Source: CAD feature listing. Evaluate the final solid. Frame: model axes, mm. A direction names the side the tool comes from. Round coordinates to 2 decimals unless told otherwise and drop trailing zeros. Order: outer loops, then holes, each group sorted by start corner. A loop starts at its lowest first (then second) coordinate and runs counter-clockwise, first axis right, second up. Notation, with made-up numbers: (51.5, 78) -> (98.5, 78) arc R20 cw to (98.5, 91) -> close; hole circle Ø3 at (-7.75, -29). An arc over 180 degrees is marked (long way). Use a Markdown table: item, result. Add a question column.
Autodesk Inventor part; units mm, degrees
ref_plane "YZ Plane" through (0, 0, 0) normal (1, 0, 0) x (0, 1, 0)
ref_plane "XZ Plane" through (0, 0, 0) normal (0, 1, 0) x (-1, 0, 0)
ref_plane "XY Plane" through (0, 0, 0) normal (0, 0, 1) x (1, 0, 0)
sketch "草圖1" plane through (0, 0, 0) normal (0, 1, 0) x (-1, 0, 0)
  line L0 (0, 0) -> (-30, 0)
  line L1 (-30, 0) -> (-30, -50)
  line L2 (-30, -50) -> (0, -50)
  line L3 (0, -50) -> (0, 0)
  line L4 (-30, -50) -> (-60, -50)
  line L5 (-60, -50) -> (-60, -30)
  line L6 (-60, -30) -> (-30, -30)
  line L7 (-30, -30) -> (-30, -50)
  dimension "d0" = 30
  dimension "d1" = 20
  dimension "d2" = 30
  dimension "d6" = 30
extrude "擠出1" add sketch "草圖1" along normal blind 10
sketch "草圖2" plane through (60, 0, -50) normal (0, 0, -1) x (-1, 0, 0)
  line L0 (60, 0) -> (60, 10)
  line L1 (60, 10) -> (40, 10)
  line L2 (40, 10) -> (40, 30)
  line L3 (40, 30) -> (60, 30)
  line L4 (60, 30) -> (60, 10)
  line L5 (40, 10) -> (10, 10)
  line L6 (10, 10) -> (10, 20)
  line L7 (10, 20) -> (40, 20)
  line L8 (40, 20) -> (40, 10)
  line L9 (10, 10) -> (0, 10)
  line L10 (0, 10) -> (0, 50)
  line L11 (0, 50) -> (10, 50)
  line L12 (10, 50) -> (10, 10)
  dimension "d7" = 10
  dimension "d8" = 30
  dimension "d9" = 20
  dimension "d10" = 20
  dimension "d11" = 10
  dimension "d12" = 40
extrude "擠出2" add sketch "草圖2" against normal blind 10
sketch "草圖3" plane through (0, 0, -50) normal (-1, 0, 0) x (0, 0, 1)
  line L0 (0, 30) -> (10, 30)
  line L1 (50, 10) -> (20, 10)
  line L2 (10, 30) -> (50, 10)
  line L3 (50, 10) -> (10, 10)
  line L4 (10, 20) -> (10, 30)
  line L5 (10, 10) -> (10, 30)
  point P0 (50, 0)
extrude "擠出3" add sketch "草圖3" against normal blind 10
fillet "圓角1" radius 10 3 edges at (60, 50, -45) (60, 5, -30) (30, 5, 0)
properties part number "5"
1) Line query: probe 1 along Y at (x, z) = (24, -27); probe 2 along Y at (x, z) = (11.5, -43.5). Output: solid intervals per line, ascending. Write a range as from..to.
2) Section D-D on y = 17. Output: boundary loops of the cut face in (x, z), then the cut area to 3 significant figures.
3) Section C-C on x = 38.5. Output: boundary loops of the cut face in (y, z), then the cut area to 3 significant figures.
4) Draft query along X for faces 4 (the flat face through (10, 16, -29)), 5 (the flat face through (10, 5, 0)), 6 (the flat face through (50, 35, -45)). Return one class per face: pulls with the +X half, pulls with the -X half, needs draft (parallel to the pull), parting line crosses it, or undercut.
5) Section A-A on y = 25. Output: boundary loops of the cut face in (x, z).
6) First-contact query: pin 1 Ø8 at (y, z) = (34.5, -45.5) entering from -X; pin 2 Ø6 at (x, y) = (29, 17) entering from +Z; pin 3 Ø10 at (y, z) = (20.5, -25.5) entering from +X. Flat tips, straight axial feed; report the tip coordinate or a pass-through.
7) Reachability of faces 1 (the flat face through (35, 20, -45)), 2 (the flat face through (41, 17, -40)), 3 (the flat face through (30, 5, -20)) from +Z, -Z, +X, -X, +Y, -Y: full face, straight path, thin tool, end or side. Return the list, or none.
Conclusion:
| question | item | result |
|---|---|---|
| 1 | probe 1 | y = 0..10 |
| 1 | probe 2 | y = 0..30 |
| 2 | outline | (0, -50) -> (60, -50) -> (60, -40) -> (10, -40) -> (10, -14) -> (0, -14) -> close |
| 2 | area | 860 mm^2 |
| 3 | outline | (0, -50) -> (20, -50) -> (20, -40) -> (10, -40) -> (10, -30) -> (0, -30) -> close |
| 3 | area | 300 mm^2 |
| 4 | face 4 | pulls with the +X half |
| 4 | face 5 | needs draft |
| 4 | face 6 | undercut |
| 5 | outline | (0, -50) -> (20, -50) -> (20, -40) -> (10, -40) -> (10, -30) -> (0, -30) -> close; (50, -50) -> (60, -50) -> (60, -40) -> (50, -40) -> close |
| 6 | pin 1 | stops at x = 50 |
| 6 | pin 2 | stops at z = -40 |
| 6 | pin 3 | stops at x = 10 |
| 7 | face 1 | +Z, -Z, +Y |
| 7 | face 2 | +Z, +X, +Y |
| 7 | face 3 | +Z, +X, +Y, -Y |
